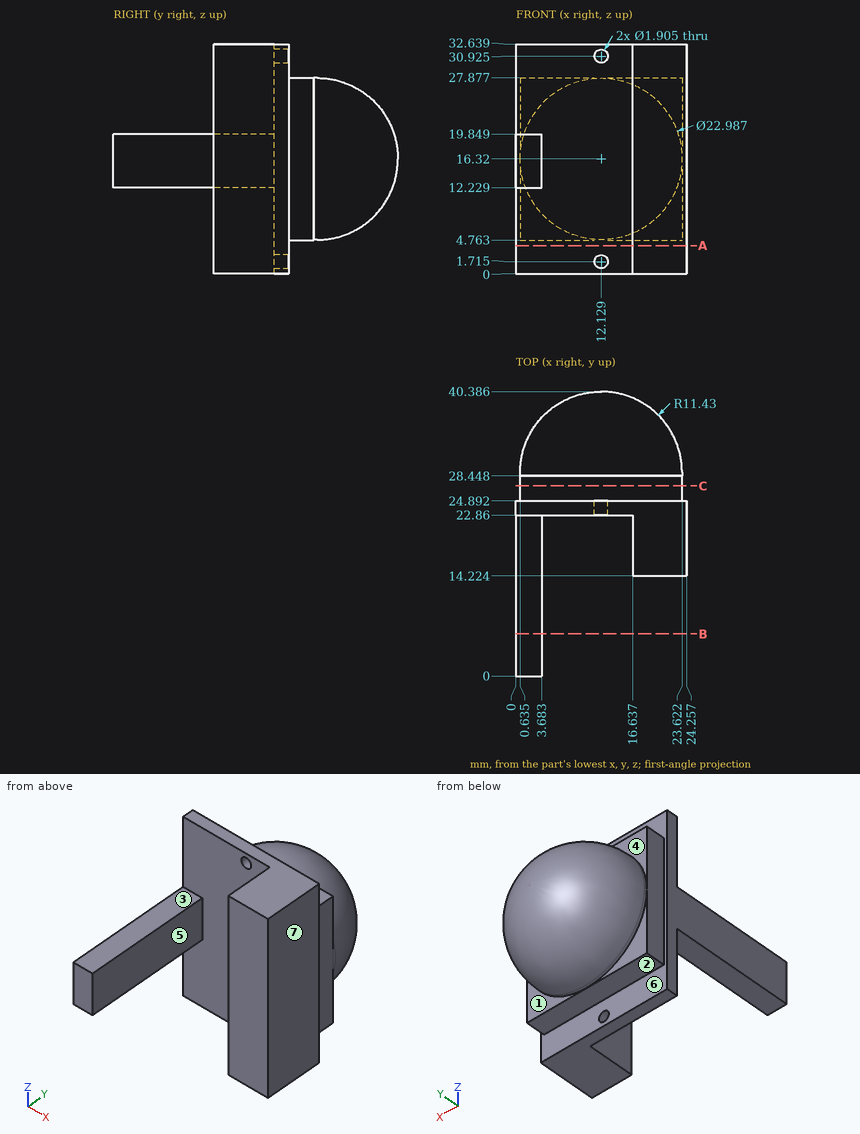
Print and shaded views of the part. All mm, measured from the part's lowest x, y and z. A direction names the side the tool comes from. Coordinates: 2 decimals unless noted, no trailing zeros. Loops run counter-clockwise (first coordinate to the right, second up) from the corner with the lowest first, then second, coordinate; pieces in that order, holes last. Notation, with made-up numbers: (-13.75, 50.25) - (-6.75, 50.25) arc R31 ccw to (-6.75, 78.25) - close; hole circle Ø4 at (-26, -36). An arc over 180 degrees is marked (long way). Write item = value, one per line. Start each with the question number.
Item 1: Cut at B-B, the plane y = 6. Give the cut face in (x, z).
Item 2: Wall check: L1, parallel to X at y = 20, z = 15.5; L2, parallel to Z at x = 16.75, y = 26.5; L3, parallel to Y at x = 18.75, z = 29.5 (1 decimal). Give the ranges that are in metal, low to high. Write a range as from..to.
Item 3: Mould opens along X. For the marked faces 5, 6 and 7 say: released by +X, released by -X, zero draft, split by the parting line, or undercut.
Item 4: Cut at C-C, the plane y = 27. Give the cut face in (x, z) (1 decimal), and give its area (3 significant figures).
Item 5: Cut at A-A, the plane z = 4. Give the cut face in (x, y) (1 decimal), and give its area (3 significant figures).
Item 6: 3-axis set-ups, long thin cutter, end or side, ignore diameter. For the marked faces 1, 2, 3 and 4: which of +Z, -Z, +X, -X, +Y, -Y reach the whole face in a straight line?
Item 7: Flat gauge pins, fed straight in: pin 1 Ø1 at (x, z) = (12, 22.5) entering from +Y; pin 2 Ø10 at (x, z) = (21.5, 17) entering from +Y; pin 3 Ø4 at (x, z) = (19.5, 10) entering from -Y; pin 4 Ø4 at (y, z) = (26, 14) entering from +X. Where does each tip first touch, or does it go through?
The answers:
q1.outline = (0, 12.23) - (3.68, 12.23) - (3.68, 19.85) - (0, 19.85) - close
q2.L1 = 0..3.68, 16.64..24.26
q2.L2 = 4.76..27.88
q2.L3 = 14.2..24.9
q3.face_5 = undercut
q3.face_6 = zero draft
q3.face_7 = released by +X
q4.outline = (0.6, 4.8) - (23.6, 4.8) - (23.6, 27.9) - (0.6, 27.9) - close
q4.area = 531 mm2
q5.outline = (0, 22.9) - (16.6, 22.9) - (16.6, 14.2) - (24.3, 14.2) - (24.3, 24.9) - (0, 24.9) - close
q5.area = 115 mm2
q6.face_1 = -Z, +Y
q6.face_2 = -Z, +X, -X, +Y
q6.face_3 = +Z, -X, -Y
q6.face_4 = +Z, +Y
q7.pin_1 = 38.91
q7.pin_2 = 39.53
q7.pin_3 = 14.22
q7.pin_4 = 24.26
